Part model, mm, in its own coordinate system. A direction names the side the tool comes from. Round coordinates to 2 decimals unless told otherwise and drop trailing zeros. Write each loop counter-clockwise with the first axis right and the second up, starting at its lowest first coordinate (ties: lowest second). Pieces come first, ordered by that corner, then holes. Notation, with made-up numbers: M 31,10 L 90,10 A14 cw 90,22 Z; hole C 22.5,-23 d6. An arc over 180 degrees is marked long. Use one line per item in the form item = value. Start each with the question number.
Item 1: Cut at A-A, the plane z = 17.75. Give the cut face in (x, y), then the cut area to 3 significant figures.
Item 2: Probe L1, parallel to X at y = 32.5, z = 11.5; L2, parallel to Y at x = 24, z = 10.5; L3, parallel to X at y = 14, z = 2.25. List the from-to ranges inside material, lowest first.
Item 3: Flat gauge pins, fed straight in: pin 1 Ø1.2 at (x, z) = (41.5, 7) entering from +Y; pin 2 Ø10 at (y, z) = (21, 6) entering from +X; pin 3 Ø12 at (y, z) = (4.5, 8) entering from -X. Where does each tip first touch, or does it go through?
Item 4: Which spindle directions (+Z, -Z, +X, -X, +Y, -Y) get a long thin tool onto all of the face, cutting with end or side? Do faces 1 (the face through (42, 10.974, 10)), 2 (the face through (-2, 10.71, 10)), 3 (the face through (40, 26, 10)), 4 (the face through (0, 26, 10)). Say none if no direction does.
Item 5: Cut at C-C, the plane y = 3.5. Give the cut face in (x, z), then the cut area to 3 significant figures.
Item 6: Cut at B-B, the plane x = 3. Give the cut face in (y, z).
Item 7: Cut at D-D, the plane z = 15. Give the cut face in (x, y), then the cut area to 3 significant figures.
from build123d import *

# Parameters (mm, degrees)
SKETCH_3_W      = 40
SKETCH_3_H      = 38.656537643
EXTRUDE_1_DEPTH = 20
SKETCH_4_R      = 7.571632933
EXTRUDE_2_DEPTH = 6
SKETCH_5_W      = 20
SKETCH_5_H      = 3.020345361
EXTRUDE_3_DEPTH = 4.002234026
SKETCH_6_W      = 20
SKETCH_6_H      = 3.435678125
EXTRUDE_4_DEPTH = 4


with BuildPart() as part:
    # 草图3 → 凸台-拉伸1 (new body)
    with BuildSketch(Plane.XY):
        with Locations((20, 19.328268822)):
            Rectangle(SKETCH_3_W, SKETCH_3_H)
    extrude(amount=EXTRUDE_1_DEPTH)

    # 草图4 → 凸台-拉伸2 (add)
    with BuildSketch(Plane(origin=(0, 0, 0), x_dir=(1, 0, 0), z_dir=(0, 1, 0))):
        with Locations(Location((9.184956981, -9.400712822, 0), (0, 0, 270))):
            Circle(SKETCH_4_R)
    extrude(amount=-EXTRUDE_2_DEPTH)

    # 草图5 → 凸台-拉伸3 (add)
    with BuildSketch(Plane.ZY):
        with Locations((10, 12.220599132)):
            Rectangle(SKETCH_5_W, SKETCH_5_H)
    extrude(amount=EXTRUDE_3_DEPTH)

    # 草图6 → 凸台-拉伸4 (add)
    with BuildSketch(Plane(origin=(40, 0, 0), x_dir=(0, 0, -1), z_dir=(1, 0, 0))):
        with Locations((-10, 12.69140217)):
            Rectangle(SKETCH_6_W, SKETCH_6_H)
    extrude(amount=EXTRUDE_4_DEPTH)


solid = part.part
Model answer:
q1.outline = M -4,10.71 L 0,10.71 L 0,0 L 40,0 L 40,10.97 L 44,10.97 L 44,14.41 L 40,14.41 L 40,38.66 L 0,38.66 L 0,13.73 L -4,13.73 Z
q1.area = 1,570 mm²
q2.L1 = 0 to 40
q2.L2 = 0 to 38.66
q2.L3 = 0 to 44
q3.pin_1 = 14.41
q3.pin_2 = 40
q3.pin_3 = 0
q4.face_1 = +Z, -Z, +X, -Y
q4.face_2 = +Z, -Z, -X, -Y
q4.face_3 = +Z, -Z, +X, +Y
q4.face_4 = +Z, -Z, -X, +Y
q5.outline = M 0,0 L 40,0 L 40,20 L 0,20 Z
q5.area = 800 mm²
q6.outline = M -6,5.03 L 0,5.03 L 0,0 L 38.66,0 L 38.66,20 L 0,20 L 0,13.77 L -6,13.77 Z
q7.outline = M -4,10.71 L 0,10.71 L 0,0 L 4.09,0 L 4.09,-6 L 14.28,-6 L 14.28,0 L 40,0 L 40,10.97 L 44,10.97 L 44,14.41 L 40,14.41 L 40,38.66 L 0,38.66 L 0,13.73 L -4,13.73 Z
q7.area = 1,630 mm²
